Source: three-view drawing plus pictorial views. Frame: mm from the lowest corner of the part. A direction names the side the tool comes from. Coordinates: 2 decimals unless noted, no trailing zeros. Order: outer loops, then holes, each group sorted by start corner. A loop starts at its lowest first (then second) coordinate and runs counter-clockwise, first axis right, second up. Notation, with made-up numbers: (52, 36.5) - (110, 36.5) arc R12 ccw to (110, 57.5) - close; hole circle Ø11 at (-2, 5.25). An arc over 180 degrees is marked (long way). Use a Markdown table: item, result. Add a question column.
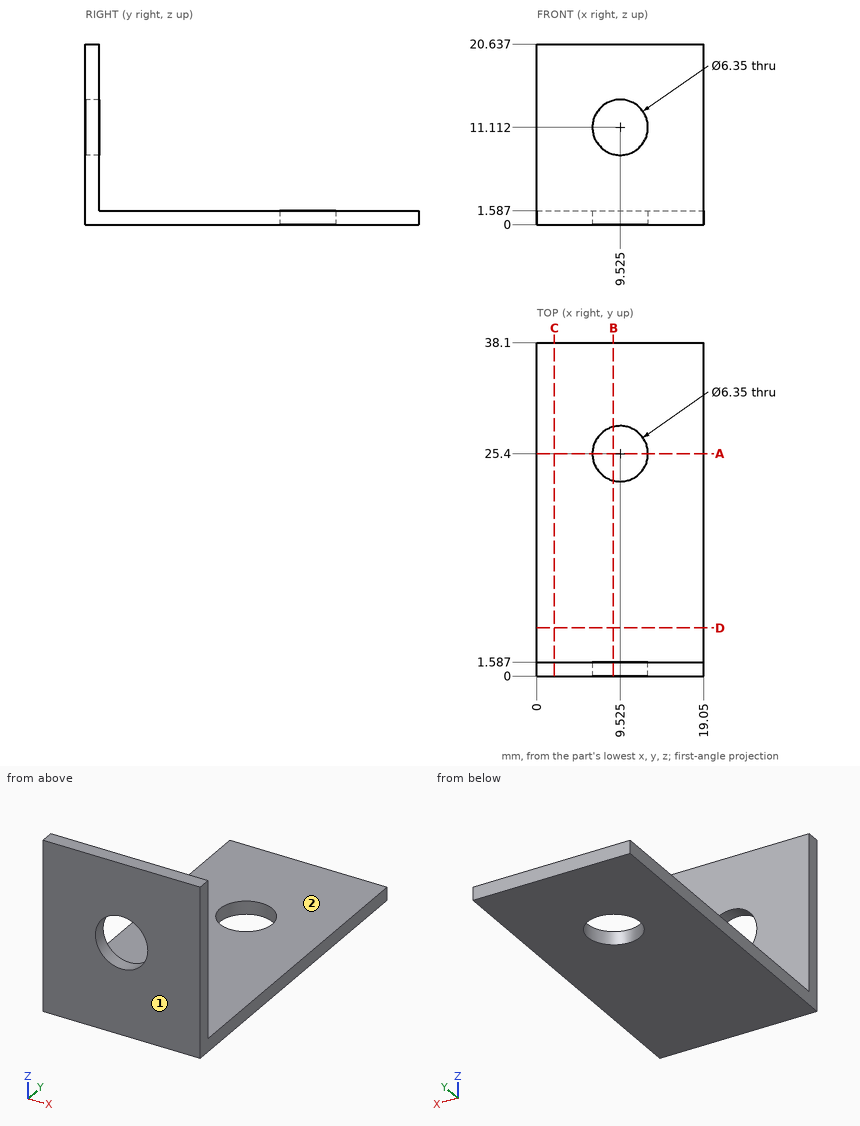
1) Ray query, line 1 along Y through (x, z) = (4.75, 4.75). Return the intervals inside material, ascending.
2) Section B-B (x = 8.75). Return loops of the section in (y, z).
3) Section A-A (y = 25.4). Return loops of the section in (x, z).
4) Set-up query: the marked faces 1 and 2. Return all of +Z, -Z, +X, -X, +Y, -Y with unobstructed straight access to the full face (end or side cutting, diameter ignored); none if empty.
5) Pin query (flat end, axial travel): pin 1 (6 mm diameter, centred on x = 14, y = 29, fed in from +Z); pin 2 (5.5 mm diameter, centred on x = 9.525, y = 25.4, fed in from +Z); pin 3 (8 mm diameter, centred on x = 15.5, z = 15.5, fed in from +Y); pin 4 (1.5 mm diameter, centred on x = 8.5, y = 14, fed in from -Z). Return the tip coordinate at first contact, or that it passes through.
6) Section D-D (y = 5.5). Return loops of the section in (x, z).
7) Section C-C (x = 2). Return loops of the section in (y, z).
Values follow:
| question | item | result |
|---|---|---|
| 1 | line 1 | y = 0 to 1.59 |
| 2 | outline | (0, 0) - (22.32, 0) - (22.32, 1.59) - (1.59, 1.59) - (1.59, 8.03) - (0, 8.03) - close; (0, 14.19) - (1.59, 14.19) - (1.59, 20.64) - (0, 20.64) - close; (28.48, 0) - (38.1, 0) - (38.1, 1.59) - (28.48, 1.59) - close |
| 3 | outline | (0, 0) - (6.35, 0) - (6.35, 1.59) - (0, 1.59) - close; (12.7, 0) - (19.05, 0) - (19.05, 1.59) - (12.7, 1.59) - close |
| 4 | face 1 | +Z, -Z, +X, -X, -Y |
| 4 | face 2 | +Z, +X, -X, +Y |
| 5 | pin 1 | stops at z = 1.59 |
| 5 | pin 2 | passes through |
| 5 | pin 3 | stops at y = 1.59 |
| 5 | pin 4 | stops at z = 0 |
| 6 | outline | (0, 0) - (19.05, 0) - (19.05, 1.59) - (0, 1.59) - close |
| 7 | outline | (0, 0) - (38.1, 0) - (38.1, 1.59) - (1.59, 1.59) - (1.59, 20.64) - (0, 20.64) - close |
